Could you check a few things on this model? Use its own coordinates, in mm. Face numbers are marked on the shaded views. Round coordinates to 2 decimals unless told otherwise and drop trailing zeros. Loops run counter-clockwise (first coordinate to the right, second up) from the corner with the lowest first, then second, coordinate; pieces in that order, holes last. Notation, with made-up numbers: M 46.25,67 L 56.25,67 A22 ccw 56.25,102 Z; hole C -21.5,57.25 d3. An arc over 180 degrees is marked long. One line per item, written item: value. Start each with the question number.
Q1. Imagine slicing it at B-B (y = -22.5). Please give me the cut outline in (x, z), then the cut area to 3 significant figures.
Q2. Please list where these lines run through material, in increasing order: line 1 along Z through (x, y) = (0, -48.5); line 2 along Z through (x, y) = (-42.5, -39.5); line 3 along X through (y, z) = (-19.5, 37.5).
Q3. Thinking about a two-plate mould opening in Z: for the marked faces 1, 2 and 3, which applies, released by +Z, released by -Z, zero draft, split by the parting line, or undercut?
Q4. I'm going to push flat-ended pins straight in: pin 1 Ø12 at (y, z) = (-42.5, 59.5) entering from -X; pin 2 Ø6 at (x, z) = (38, 77) entering from +Y; pin 3 Ø1.5 at (y, z) = (-60, 73.5) entering from +X. Where does each tip first touch, or does it pass through?
Q5. Imagine slicing it at A-A (x = 0). Please give me the cut outline in (y, z), then the cut area to 3 significant figures.
Q6. Imagine slicing it at C-C (z = 0). Please give me the cut outline in (x, y).
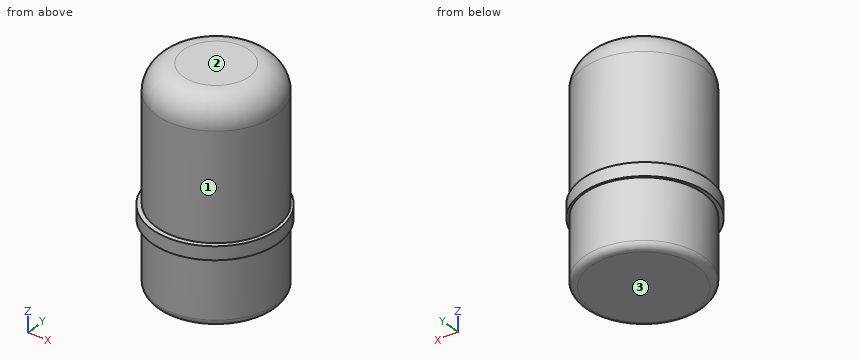
from build123d import *

# Parameters (mm, degrees)
SKETCH1_W   = 45
SKETCH1_H   = 100
SKETCH1_6_W = 47.5
SKETCH1_6_H = 10
SKETCH1_7_W = 45
SKETCH1_7_H = 50
FILLET1_R   = 20
FILLET2_R   = 5


with BuildPart() as part:
    # Sketch1 → Revolve2 (revolve)
    with BuildSketch(Plane.YZ):
        with Locations((0, 55)):
            Rectangle(SKETCH1_W, SKETCH1_H)
    revolve(axis=Axis((0, -22.5, 5), (0, 0, 1)))

    # Sketch1_6 → Revolve3 (revolve)
    with BuildSketch(Plane.YZ):
        Rectangle(SKETCH1_6_W, SKETCH1_6_H)
    revolve(axis=Axis((0, -23.75, -5), (0, 0, 1)))

    # Sketch1_7 → Revolve4 (revolve)
    with BuildSketch(Plane.YZ):
        with Locations((0, -30)):
            Rectangle(SKETCH1_7_W, SKETCH1_7_H)
    revolve(axis=Axis((0, -22.5, -55), (0, 0, 1)))

    # Fillet1
    fillet1_edges = [part.edges().sort_by_distance(p)[0] for p in [
        (0, -67.5, 105),
    ]]
    fillet(fillet1_edges, radius=FILLET1_R)

    # Fillet2
    fillet2_edges = [part.edges().sort_by_distance(p)[0] for p in [
        (0, -67.5, -55),
    ]]
    fillet(fillet2_edges, radius=FILLET2_R)


solid = part.part
Report:
1. outline: M -47.48,-5 L -45,-5 L -45,-50 A5 ccw -40,-55 L 40,-55 A5 ccw 45,-50 L 45,-5 L 47.48,-5 L 47.48,5 L 45,5 L 45,85 A20 ccw 25,105 L -25,105 A20 ccw -45,85 L -45,5 L -47.48,5 Z
1. area: 14,300 mm²
2. line 1: z = -55 to 104.97
2. line 2: z = -5 to 5
2. line 3: x = -44.9 to 44.9
3. face 1: zero draft
3. face 2: released by +Z
3. face 3: released by -Z
4. pin 1: stops at x = -42.77
4. pin 2: stops at y = 5.78
4. pin 3: stops at x = 25.97
5. outline: M -71.25,-5 L -67.5,-5 L -67.5,-50 A5 ccw -62.5,-55 L 17.5,-55 A5 ccw 22.5,-50 L 22.5,-5 L 23.75,-5 L 23.75,5 L 22.5,5 L 22.5,85 A20 ccw 2.5,105 L -47.5,105 A20 ccw -67.5,85 L -67.5,5 L -71.25,5 Z
5. area: 14,300 mm²
6. outline: C 0,-23.75 d95
